Part model, mm, in its own coordinate system. A direction names the side the tool comes from. Give positions to 0.01 mm unless a question says otherwise; leave off trailing zeros. Write each loop counter-clockwise with the first axis right and the second up, starting at its lowest first coordinate (ties: lowest second). Pieces come first, ordered by that corner, then holes. Notation, with made-up numbers: (86, 25.5) - (132, 25.5) arc R15 cw to (132, 40.5) - close; hole circle Ø11 at (38.25, 29). An arc over 180 degrees is marked (long way). Answer as a JSON object with one key per item and string values. Group by question number.
```python
from build123d import *

# Parameters (mm, degrees)
F0_W     = 44.45
F0_H     = 76.2
F1_DEPTH = 6.35
F2_W     = 6.35
F2_H     = 76.2
F3_DEPTH = 19.05
F4_R     = 3.3782
F5_DEPTH = 12.7
F7_DEPTH = 25.4


with BuildPart() as f1:
    # F0 (on Top) → F1 (new body)
    with BuildSketch(Plane.XY):
        with Locations((-75.31851, 26.558877)):
            Rectangle(F0_W, F0_H)
    extrude(amount=F1_DEPTH)

    # F2 (on face) → F3 (join)
    with BuildSketch(Plane(origin=(0, 0, 0), x_dir=(1, 0, 0), z_dir=(0, 0, -1))):
        with Locations((-94.36851, -26.558877)):
            Rectangle(F2_W, F2_H)
    extrude(amount=F3_DEPTH)

    # F4 (on face) → F5 (cut)
    with BuildSketch(Plane(origin=(-97.54351, 0, 0), x_dir=(0, -1, 0), z_dir=(-1, 0, 0))):
        with Locations((-2.555877, -7.5438)):
            Circle(F4_R)
        with Locations((-50.561877, -7.5438)):
            Circle(F4_R)
    extrude(amount=-F5_DEPTH, mode=Mode.SUBTRACT)

    # F6 (on face) → F7 (cut)
    with BuildSketch(Plane(origin=(0, 0, 0), x_dir=(1, 0, 0), z_dir=(0, 0, -1))):
        with BuildLine():
            ThreePointArc((-83.57351, -16.240127), (-82.450978, -15.775159), (-81.98601, -14.652627))
            Line((-81.98601, -14.652627), (-83.57351, -14.652627))
            Line((-83.57351, -14.652627), (-83.57351, -16.240127))
        make_face()
        with BuildLine():
            Line((-83.57351, -14.652627), (-81.98601, -14.652627))
            ThreePointArc((-81.98601, -14.652627), (-84.696042, -13.530094), (-83.57351, -16.240127))
            Line((-83.57351, -16.240127), (-83.57351, -14.652627))
        make_face()
        with BuildLine():
            Line((-59.76101, -14.652627), (-61.34851, -14.652627))
            ThreePointArc((-61.34851, -14.652627), (-60.883542, -15.775159), (-59.76101, -16.240127))
            Line((-59.76101, -16.240127), (-59.76101, -14.652627))
        make_face()
        with BuildLine():
            ThreePointArc((-58.17351, -14.652627), (-59.76101, -13.065127), (-61.34851, -14.652627))
            Line((-61.34851, -14.652627), (-59.76101, -14.652627))
            Line((-59.76101, -14.652627), (-59.76101, -16.240127))
            ThreePointArc((-59.76101, -16.240127), (-58.638478, -15.775159), (-58.17351, -14.652627))
        make_face()
        with BuildLine():
            Line((-83.57351, -38.465127), (-83.57351, -36.877627))
            ThreePointArc((-83.57351, -36.877627), (-84.696042, -39.587659), (-81.98601, -38.465127))
            Line((-81.98601, -38.465127), (-83.57351, -38.465127))
        make_face()
        with BuildLine():
            ThreePointArc((-81.98601, -38.465127), (-82.450978, -37.342594), (-83.57351, -36.877627))
            Line((-83.57351, -36.877627), (-83.57351, -38.465127))
            Line((-83.57351, -38.465127), (-81.98601, -38.465127))
        make_face()
        with BuildLine():
            ThreePointArc((-58.17351, -38.465127), (-58.638478, -37.342594), (-59.76101, -36.877627))
            Line((-59.76101, -36.877627), (-59.76101, -38.465127))
            Line((-59.76101, -38.465127), (-61.34851, -38.465127))
            ThreePointArc((-61.34851, -38.465127), (-59.76101, -40.052627), (-58.17351, -38.465127))
        make_face()
        with BuildLine():
            Line((-59.76101, -38.465127), (-59.76101, -36.877627))
            ThreePointArc((-59.76101, -36.877627), (-60.883542, -37.342594), (-61.34851, -38.465127))
            Line((-61.34851, -38.465127), (-59.76101, -38.465127))
        make_face()
    extrude(amount=-F7_DEPTH, mode=Mode.SUBTRACT)


solid = f1.part
```
1) Saw through at D-D (y = 33.5). List the corners of the cut face in (x, z).
2) Drill centre lines: line 1 along Z through (x, y) = (-69.5, 48.5); line 2 along X through (y, z) = (3, -11.75). Where is each one in solid material? Low to high. Write a range as from..to.
3) Two-plate mould, pull along Z, no slides. Class faces 1 (the flat face through (-80.4, 64.659, 0.3)), 2 (the flat face through (-72, 27, 0)), 3 (the cylindrical face through (-94.413, 2.996, -4.194)): +Z half, -Z half, draft (parallel to the pull), parting line (faces both ways), or undercut.
4) Saw through at B-B (x = -60.5). List the corners of the cut face in (y, z).
5) Which spindle directions (+Z, -Z, +X, -X, +Y, -Y) get a long thin tool onto all of the face, cutting with end or side? Do faces 4 (the flat face through (-91.194, 27, -9)), 5 (the flat face through (-53.094, 26, 3)). Say none if no direction does.
6) Saw through at C-C (z = -5.5). List the corners of the cut face in (x, y).
7) Drop flat-ended pins along their axis: P1, Ø8, axis at x = -86, y = 29, coming from the -Z side; P2, Ø15, axis at y = 45, z = -12.5, coming from the +X side; P3, Ø4, axis at y = 2.56, z = -7.54, coming from the -X side. Give the stop position or say it passes through.
8) Saw through at A-A (y = 50). List the corners of the cut face in (x, z), and give its area (3 significant figures).
Checks:
{
 "1": {"outline": "(-97.54, -19.05) - (-91.19, -19.05) - (-91.19, 0) - (-53.09, 0) - (-53.09, 6.35) - (-97.54, 6.35) - close"},
 "2": {"line 1": "0..6.35", "line 2": "-97.54..-91.19"},
 "3": {"face 1": "draft", "face 2": "-Z half", "face 3": "undercut"},
 "4": {"outline": "(-11.54, 0) - (13.25, 0) - (13.25, 6.35) - (-11.54, 6.35) - close; (16.06, 0) - (37.06, 0) - (37.06, 6.35) - (16.06, 6.35) - close; (39.87, 0) - (64.66, 0) - (64.66, 6.35) - (39.87, 6.35) - close"},
 "5": {"face 4": "-Z, +X, +Y, -Y", "face 5": "+Z, -Z, +X, +Y, -Y"},
 "6": {"outline": "(-97.54, -11.54) - (-91.19, -11.54) - (-91.19, -0.13) - (-97.54, -0.13) - close; (-97.54, 5.25) - (-91.19, 5.25) - (-91.19, 47.87) - (-97.54, 47.87) - close; (-97.54, 53.25) - (-91.19, 53.25) - (-91.19, 64.66) - (-97.54, 64.66) - close"},
 "7": {"P1": "z = 0", "P2": "x = -91.19", "P3": "through"},
 "8": {"outline": "(-97.54, -19.05) - (-91.19, -19.05) - (-91.19, -10.87) - (-97.54, -10.87) - close; (-97.54, -4.21) - (-91.19, -4.21) - (-91.19, 0) - (-53.09, 0) - (-53.09, 6.35) - (-97.54, 6.35) - close", "area": "361 mm2"}
}
